```python
from build123d import *

# Parameters (mm, degrees)
SKETCH1_R             = 4
BOSS_EXTRUDE1_DEPTH   = 5
BODY_MOVE_COPY1_ANGLE = 90


with BuildPart() as part:
    # Sketch1 → Boss-Extrude1 (new body)
    with BuildSketch(Plane(origin=(0, 0, 0), x_dir=(1, 0, 0), z_dir=(0, 1, 0))):
        with BuildLine():
            Line((13.747727104, -9.999999956), (186.252272934, -9.999999956))
            ThreePointArc((186.252272934, -9.999999956), (189.598913044, -8.190890181), (189.918333485, -4.399999944))
            ThreePointArc((189.918333485, -4.399999944), (202.569546944, 10.695673442), (206.982653657, -8.499561542))
            Line((206.982653657, -8.499561542), (193.869713288, -19.272249007))
            ThreePointArc((193.869713288, -19.272249007), (190.297826985, -21.297499344), (186.252273428, -21.999999956))
            Line((186.252273428, -21.999999956), (13.747727597, -21.999999956))
            ThreePointArc((13.747727597, -21.999999956), (9.702173549, -21.297499522), (6.130286801, -19.272249048))
            Line((6.130286801, -19.272249048), (-6.982653611, -8.499561668))
            ThreePointArc((-6.982653611, -8.499561668), (-2.569547007, 10.695673339), (10.081666543, -4.399999968))
            ThreePointArc((10.081666543, -4.399999968), (10.401087001, -8.190890191), (13.747727104, -9.999999956))
        make_face()
        Circle(SKETCH1_R, mode=Mode.SUBTRACT)
        with Locations((200, 8.8e-08)):
            Circle(SKETCH1_R, mode=Mode.SUBTRACT)
    extrude(amount=BOSS_EXTRUDE1_DEPTH)


with BuildPart() as part_1:
    # Body-Move/Copy1: moved
    add(part.part.moved(Location((0, 0, 0))).rotate(Axis((100, 2.5, 0), (0, 0, 1)), BODY_MOVE_COPY1_ANGLE))


solid = part_1.part
```
Model file for the job. Use its own axes, mm. A direction names the side the tool comes from. Coordinates: 2 decimals unless noted, no trailing zeros. Write each loop counter-clockwise with the first axis right and the second up, starting at its lowest first coordinate (ties: lowest second). Pieces come first, ordered by that corner, then holes. Notation, with made-up numbers: (18, 65) - (56, 65) arc R32 cw to (56, 91) - close; hole circle Ø3 at (17.5, -3.5). An arc over 180 degrees is marked (long way). One line per item, written item: value. Start each with the question number.
1. Flat gauge pin, fed straight in: pin 1 (2 mm diameter, centred on x = 101, y = 84, fed in from -Z). Where does the tip first touch, or does it go through?
2. Mould opens along Y. For faces 3 (the cylindrical face through (100.035, 92.068, 8.237)), 4 (the flat face through (100.04, 103.02, 13.81)), 5 (the cylindrical face through (100.03, -87.13, 8.14)), 6 (the flat face through (102.5, 4, 13)) say: released by +Y, released by -Y, zero draft, split by the parting line, or undercut.
3. Tool access for faces 1 (the cylindrical face through (100.04, 104.74, -10.77)), 2 (the flat face through (100, 1, 10)): list every direction of +Z, -Z, +X, -X, +Y, -Y with a clear straight run to the whole face (end or side of a thin tool).
4. Slice it at D-D (y = 37.5). Write the cut outline in (x, z), plus the area to 3 significant figures.
5. Slice it at C-C (y = 102.5). Write the cut outline in (x, z).
6. Slice it at B-B (x = 100.55). Write the cut outline in (y, z).
7. Probe line 1 (Y direction, x = 101.4, z = 0); line 2 (Y direction, x = 100.7, z = 1); line 3 (Z direction, x = 99.65, y = -14). List the from-to ranges inside material, lowest first. Write a range as from..to.
8. Slice it at A-A (z = 0). Write the cut outline in (x, y), plus the area to 3 significant figures.
Answers below:
1. pin 1: stops at z = 10
2. face 3: undercut
2. face 4: released by +Y
2. face 5: undercut
2. face 6: zero draft
3. face 1: +X, -X
3. face 2: -Z, +X, -X
4. outline: (97.5, 10) - (102.5, 10) - (102.5, 22) - (97.5, 22) - close
4. area: 60.0 mm^2
5. outline: (97.5, -11) - (102.5, -11) - (102.5, -4) - (97.5, -4) - close; (97.5, 4) - (102.5, 4) - (102.5, 14.24) - (97.5, 14.24) - close
6. outline: (-104.48, 8.5) arc R11 ccw (long way) to (-87.42, 4.4) arc R4 cw to (-83.75, 10) - (88.75, 10) arc R4 cw to (92.42, 4.4) arc R11 ccw (long way) to (109.48, 8.5) - (96.37, 19.27) arc R12 ccw to (88.75, 22) - (-83.75, 22) arc R12 ccw to (-91.37, 19.27) - close; hole circle Ø8 at (-97.5, 0); hole circle Ø8 at (102.5, 0)
7. line 1: y = -108.5..-101.5, -93.5..-86.5, 91.5..98.5, 106.5..113.5
7. line 2: y = -108.45..-101.37, -93.63..-86.55, 91.55..98.63, 106.37..113.45
7. line 3: z = 10..22
8. outline: (97.5, -108.5) - (102.5, -108.5) - (102.5, -101.5) - (97.5, -101.5) - close; (97.5, -93.5) - (102.5, -93.5) - (102.5, -86.5) - (97.5, -86.5) - close; (97.5, 91.5) - (102.5, 91.5) - (102.5, 98.5) - (97.5, 98.5) - close; (97.5, 106.5) - (102.5, 106.5) - (102.5, 113.5) - (97.5, 113.5) - close
8. area: 140 mm^2
